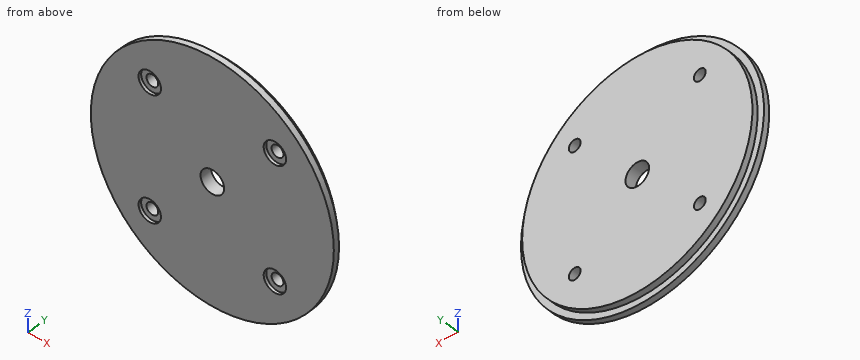
from build123d import *

# Parameters (mm, degrees)
SKETCH2_R                   = 65.405
BOSS_EXTRUDE1_DEPTH         = 6.35
SKETCH4_R                   = 65.405
SKETCH4_R_2                 = 61.976
CUT_EXTRUDE1_DEPTH          = 3.175
F_1_4_0_25_DIAMETER_HOLE1_D = 6.35
F_1_2_0_5_DIAMETER_HOLE1_D  = 12.7
SKETCH9_R                   = 6.0325
CUT_EXTRUDE2_DEPTH          = 1.5875


with BuildPart() as part:
    # Sketch2 → Boss-Extrude1 (new body)
    with BuildSketch(Plane(origin=(0, 0, 0), x_dir=(1, 0, 0), z_dir=(0, 1, 0))):
        Circle(SKETCH2_R)
    extrude(amount=BOSS_EXTRUDE1_DEPTH)

    # Sketch4 → Cut-Extrude1 (cut)
    with BuildSketch(Plane(origin=(0, 6.35, 0), x_dir=(1, 0, 0), z_dir=(0, 1, 0))):
        Circle(SKETCH4_R)
        Circle(SKETCH4_R_2, mode=Mode.SUBTRACT)
    extrude(amount=-CUT_EXTRUDE1_DEPTH, mode=Mode.SUBTRACT)

    # 1/4 (0.25) Diameter Hole1 (through all)
    with Locations(Plane(origin=(0, 6.35, 0), x_dir=(1, 0, 0), z_dir=(0, 1, 0))):
        with Locations((-33.675960454, 33.675960454), (-33.675960454, -33.675960454), (33.675960454, 33.675960454), (33.675960454, -33.675960454)):
            Hole(F_1_4_0_25_DIAMETER_HOLE1_D / 2)

    # 1/2 (0.5) Diameter Hole1 (through all)
    with Locations(Plane(origin=(0, 6.35, 0), x_dir=(1, 0, 0), z_dir=(0, 1, 0))):
        with Locations((0, 0)):
            Hole(F_1_2_0_5_DIAMETER_HOLE1_D / 2)

    # Sketch9 → Cut-Extrude2 (cut)
    with BuildSketch(Plane.XZ):
        with Locations((-33.675960454, 33.675960454)):
            Circle(SKETCH9_R)
        with Locations((33.675960454, 33.675960454)):
            Circle(SKETCH9_R)
        with Locations((33.675960454, -33.675960454)):
            Circle(SKETCH9_R)
        with Locations((-33.675960454, -33.675960454)):
            Circle(SKETCH9_R)
    extrude(amount=-CUT_EXTRUDE2_DEPTH, mode=Mode.SUBTRACT)


solid = part.part
CAD build for the part. Positions are in the model's coordinates, mm. Give positions to 0.01 mm unless a question says otherwise; leave off trailing zeros. Order: outer loops, then holes, each group sorted by start corner. A loop starts at its lowest first (then second) coordinate and runs counter-clockwise, first axis right, second up. Notation, with made-up numbers: (80.25, 62) - (95.25, 62) arc R13 ccw to (95.25, 84) - close; hole circle Ø8 at (67, -29.5). An arc over 180 degrees is marked (long way). Answer in a Markdown table with one row per item.
1. Probe probe 1 along X at (y, z) = (0.5, -38); probe 2 along Z at (x, y) = (-29, 0.75); probe 3 along X at (y, z) = (0.5, -29.5). List the from-to ranges inside material, lowest first. Write a range as [from, to].
Data:
| item | result |
|---|---|
| probe 1 | x = [-53.23, -37.88], [-29.47, 29.47], [37.88, 53.23] |
| probe 2 | z = [-58.62, -37.49], [-29.86, 29.86], [37.49, 58.62] |
| probe 3 | x = [-58.37, -38.03], [-29.32, 29.32], [38.03, 58.37] |
2. Saw through at C-C, the plane z = -17. Give the cut face in (x, y) (3 decimals).
Data:
| item | result |
|---|---|
| outline | (-63.157, 0) - (63.157, 0) - (63.157, 3.175) - (59.599, 3.175) - (59.599, 6.35) - (-59.599, 6.35) - (-59.599, 3.175) - (-63.157, 3.175) - close |
3. Saw through at B-B, the plane x = 0. Give the cut face in (y, z) (3 decimals), plus the area to 3 significant figures.
Data:
| item | result |
|---|---|
| outline | (0, -65.405) - (3.175, -65.405) - (3.175, -61.976) - (6.35, -61.976) - (6.35, -6.35) - (0, -6.35) - close; (0, 6.35) - (6.35, 6.35) - (6.35, 61.976) - (3.175, 61.976) - (3.175, 65.405) - (0, 65.405) - close |
| area | 728 mm² |
4. Flat gauge pins, fed straight in: pin 1 (6 mm diameter, centred on x = 35.5, z = -35.5, fed in from -Y); pin 2 (5.5 mm diameter, centred on x = 33.68, z = -33.68, fed in from +Y); pin 3 (3 mm diameter, centred on y = 4.5, z = -26.5, fed in from -X); pin 4 (3 mm diameter, centred on y = 3.5, z = 50, fed in from +X). Where does each tip first touch, or does it go through?
Data:
| item | result |
|---|---|
| pin 1 | stops at y = 1.59 |
| pin 2 | passes through |
| pin 3 | stops at x = -60.1 |
| pin 4 | stops at x = 43.84 |
5. Saw through at A-A, the plane z = 0. Give the cut face in (x, y) (3 decimals).
Data:
| item | result |
|---|---|
| outline | (-65.405, 0) - (-6.35, 0) - (-6.35, 6.35) - (-61.976, 6.35) - (-61.976, 3.175) - (-65.405, 3.175) - close; (6.35, 0) - (65.405, 0) - (65.405, 3.175) - (61.976, 3.175) - (61.976, 6.35) - (6.35, 6.35) - close |
6. Saw through at D-D, the plane x = 18.5. Give the cut face in (y, z) (3 decimals).
Data:
| item | result |
|---|---|
| outline | (0, -62.734) - (3.175, -62.734) - (3.175, -59.15) - (6.35, -59.15) - (6.35, 59.15) - (3.175, 59.15) - (3.175, 62.734) - (0, 62.734) - close |
